from build123d import *

# Parameters (mm, degrees)
CROQUIS1_W              = 12
CROQUIS1_H              = 20
CROQUIS1_R              = 2.5
SALIENTE_EXTRUIR1_DEPTH = 1
CROQUIS2_W              = 12
CROQUIS2_H              = 1
SALIENTE_EXTRUIR2_DEPTH = 16
CROQUIS3_R              = 2.5
CORTAR_EXTRUIR1_DEPTH   = 8
REDONDEO2_R             = 1
REDONDEO3_R             = 2


with BuildPart() as part:
    # Croquis1 → Saliente-Extruir1 (new body)
    with BuildSketch(Plane.XY):
        with Locations((0, -10)):
            Rectangle(CROQUIS1_W, CROQUIS1_H)
        with Locations((0, -12)):
            Circle(CROQUIS1_R, mode=Mode.SUBTRACT)
    extrude(amount=SALIENTE_EXTRUIR1_DEPTH)

    # Croquis2 → Saliente-Extruir2 (add)
    with BuildSketch(Plane.XY.offset(1)):
        with Locations((0, -0.5)):
            Rectangle(CROQUIS2_W, CROQUIS2_H)
    extrude(amount=SALIENTE_EXTRUIR2_DEPTH)

    # Croquis3 → Cortar-Extruir1 (cut)
    with BuildSketch(Plane.XZ.offset(1)):
        with Locations(Location((0, 9, 0), (0, 0, 270))):
            Circle(CROQUIS3_R)
    extrude(amount=-CORTAR_EXTRUIR1_DEPTH, mode=Mode.SUBTRACT)

    # Redondeo2
    redondeo2_edges = [part.edges().sort_by_distance(p)[0] for p in [
        (0, -1, 1),
    ]]
    fillet(redondeo2_edges, radius=REDONDEO2_R)

    # Redondeo3
    redondeo3_edges = [part.edges().sort_by_distance(p)[0] for p in [
        (0, 0, 0),
    ]]
    fillet(redondeo3_edges, radius=REDONDEO3_R)


solid = part.part
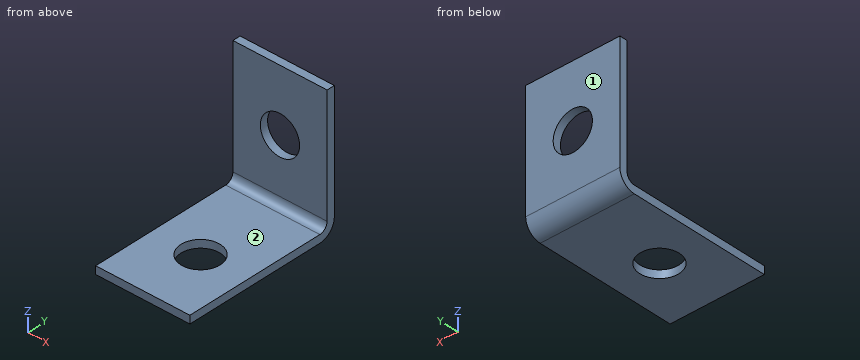
Geometry: final body of the model. Coordinates: model frame, mm. Face numbers are marked on the shaded views. A direction names the side the tool comes from. Coordinates: 2 decimals unless noted, no trailing zeros. Order: outer loops, then holes, each group sorted by start corner. A loop starts at its lowest first (then second) coordinate and runs counter-clockwise, first axis right, second up.
(1) First-contact query: pin 1 (1 mm diameter, centred on x = 3, z = 11.5, fed in from -Y). Flat tip, straight axial feed; report the tip coordinate or a pass-through.
(2) Access query for the marked faces 1 and 2. Directions: +Z, -Z, +X, -X, +Y, -Y. A direction counts if a zero-diameter tool reaches every point of the face in a straight line with its end or side. Return the directions, or none.
(3) Section query D-D (x = -4.25). Return the cut outline in (y, z), plus the area to 3 significant figures.
(4) Section query B-B (z = 9). Return the cut outline in (x, y), plus the area to 3 significant figures.
(5) Section query C-C (x = 0). Return the cut outline in (y, z).
(6) Material intervals for probe 1 along X at (y, z) = (-0.6, 9); probe 2 along Y at (x, z) = (3.5, 2.5); probe 3 along Z at (x, y) = (-2.5, -5.5), sorted ascending.
(7) Section query A-A (y = -12). Return the cut outline in (x, z).
Solution:
1. pin 1: stops at y = -1
2. face 1: +Z, -Z, +X, -X, +Y
2. face 2: +Z, +X, -X, -Y
3. outline: (-20, 0) - (-2, 0) arc R2 ccw to (0, 2) - (0, 17) - (-1, 17) - (-1, 2) arc R1 cw to (-2, 1) - (-20, 1) - close
3. area: 35.4 mm2
4. outline: (-6, -1) - (-2.5, -1) - (-2.5, 0) - (-6, 0) - close; (2.5, -1) - (6, -1) - (6, 0) - (2.5, 0) - close
4. area: 7.00 mm2
5. outline: (-20, 0) - (-14.5, 0) - (-14.5, 1) - (-20, 1) - close; (-9.5, 0) - (-2, 0) arc R2 ccw to (0, 2) - (0, 6.5) - (-1, 6.5) - (-1, 2) arc R1 cw to (-2, 1) - (-9.5, 1) - close; (-1, 11.5) - (0, 11.5) - (0, 17) - (-1, 17) - close
6. probe 1: x = -6 to -2.5, 2.5 to 6
6. probe 2: y = -1 to 0
6. probe 3: z = 0 to 1
7. outline: (-6, 0) - (-2.5, 0) - (-2.5, 1) - (-6, 1) - close; (2.5, 0) - (6, 0) - (6, 1) - (2.5, 1) - close
